Read the model definition and answer for the solid it produces. Units are mm, in the model's axes. Face numbers are marked on the shaded views. Give positions to 0.01 mm unless a question says otherwise; leave off trailing zeros. Order: outer loops, then holes, each group sorted by start corner. A loop starts at its lowest first (then second) coordinate and runs counter-clockwise, first axis right, second up. Notation, with made-up numbers: (41.5, 40) -> (67.5, 40) arc R23 cw to (67.5, 73) -> close; hole circle Ø1 at (33, -39.75). An arc over 180 degrees is marked (long way). Use one line per item in the form item = value.
```python
from build123d import *

# Parameters (mm, degrees)
SKETCH006_R       = 4
EXTRUDE008_DEPTH  = 13
CYLINDER003_R     = 43
CYLINDER003_DEPTH = 13
CYLINDER002_R     = 44
CYLINDER002_DEPTH = 13


with BuildPart() as extrude008:
    # Sketch006 → Extrude008 (new body)
    with BuildSketch(Plane.XY):
        with Locations((-5.45, 39.43)):
            Circle(SKETCH006_R)
    extrude(amount=EXTRUDE008_DEPTH)


with BuildPart() as extrude008_1:
    # Extrude008 placement: moved
    add(extrude008.part.moved(Location((0, 0, -5))))


with BuildPart() as overlap_cutout:
    # Cylinder003 → Cylinder003 (new body)
    with BuildSketch(Plane.XY.offset(-5)):
        Circle(CYLINDER003_R)
    extrude(amount=CYLINDER003_DEPTH)

    # Fusion: union Extrude008
    add(extrude008_1.part)


with BuildPart() as overlap_with_cutout:
    # Cylinder002 → Cylinder002 (new body)
    with BuildSketch(Plane.XY.offset(-5)):
        Circle(CYLINDER002_R)
    extrude(amount=CYLINDER002_DEPTH)

    # Cut006: cut overlap-cutout
    add(overlap_cutout.part, mode=Mode.SUBTRACT)


solid = overlap_with_cutout.part
```
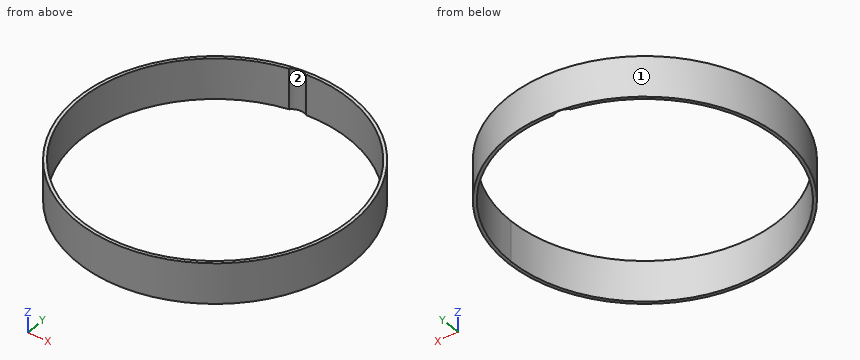
Item 1: Determine the mould class of the marked faces 1 and 2 for opening direction Y: +Y half, -Y half, draft (parallel to the pull), parting line (faces both ways), or undercut.
Checks:
face_1 = parting line
face_2 = undercut
Item 2: The part is cut by section C-C on z = 3.25. Give the vertices of the cut face in (x, y), and give its area (3 significant figures).
Checks:
outline = circle Ø88 at (0, 0); hole (-8.35, 42.18) arc R43 ccw (long way) to (-3.4, 42.87) arc R4 ccw to start
area = 271 mm²
Item 3: The part is cut by section A-A on x = 0. Give the vertices of the cut face in (y, z), and give its area (3 significant figures).
Checks:
outline = (-44, -5) -> (-43, -5) -> (-43, 8) -> (-44, 8) -> close; (43, -5) -> (44, -5) -> (44, 8) -> (43, 8) -> close
area = 26.0 mm²
Item 4: Straight lines are drawn through the part: L1, parallel to Y at x = 0, z = -1.75; L2, parallel to X at y = 6, z = 6; L3, parallel to X at y = -19.5, z = 3. For each, find the intervals that lie inside material, in ascending order. Write a range as from..to.
Checks:
L1 = -44..-43, 43..44
L2 = -43.59..-42.58, 42.58..43.59
L3 = -39.44..-38.32, 38.32..39.44
Item 5: The part is cut by section B-B on y = 16.5. Give the vertices of the cut face in (x, z).
Checks:
outline = (-40.79, -5) -> (-39.71, -5) -> (-39.71, 8) -> (-40.79, 8) -> close; (39.71, -5) -> (40.79, -5) -> (40.79, 8) -> (39.71, 8) -> close
Item 6: Given pin 1 Ø1.5 at (y, z) = (-23, 0) entering from -X; pin 2 Ø1 at (x, z) = (23, -2.5) entering from +Y; pin 3 Ø1 at (x, z) = (32, 5) entering from -Y, each flat-ended and moving along its own axis, determine where each tip first touches the part or whether it passes through.
Checks:
pin_1 = -37.96
pin_2 = 37.81
pin_3 = -30.72
